The figure shows three views and two pictorial views of one solid part (mm, origin at its lowest corner). Answer the questions. A direction names the side the tool comes from. Round coordinates to 2 decimals unless told otherwise and drop trailing zeros. Order: outer loops, then holes, each group sorted by start corner. A loop starts at its lowest first (then second) coordinate and runs counter-clockwise, first axis right, second up. Notation, with made-up numbers: M 88.25,19.25 L 118.25,19.25 A3 ccw 118.25,23.25 Z; hole C 68,61.25 d1. An arc over 180 degrees is marked long. Return JSON: item names as keys, results as strings.
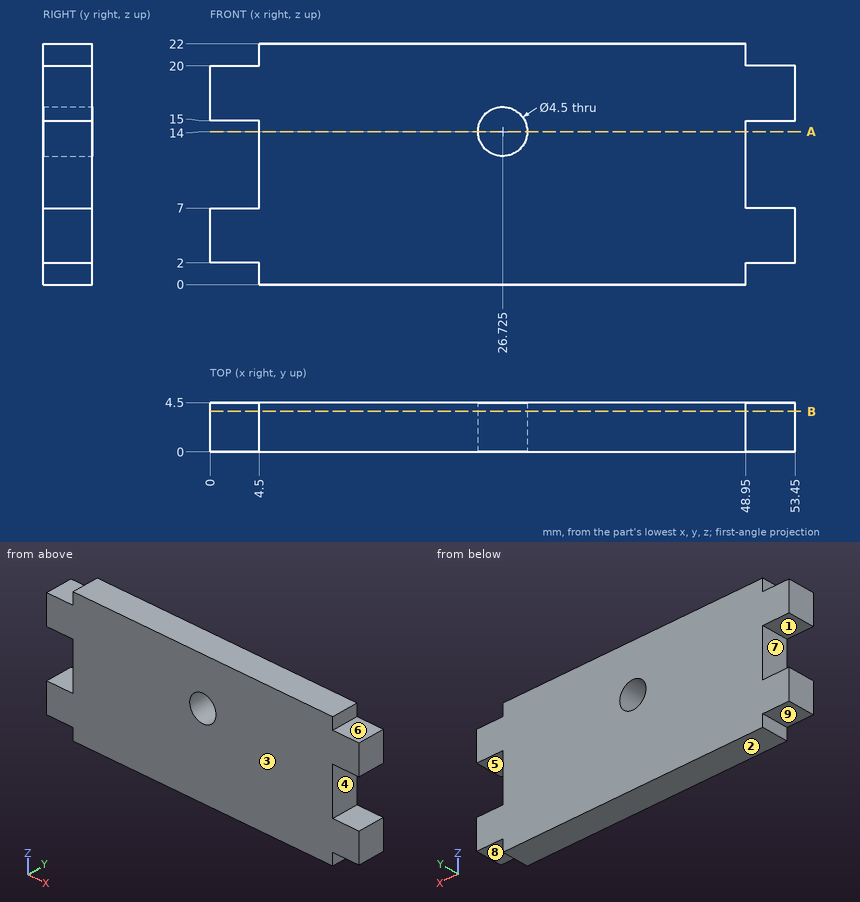
Item 1: Each of these flat-tipped pins is pushed along its axis until it touches: pin 1 (2 mm diameter, centred on x = 51.5, y = 3.5, fed in from -Z); pin 2 (0.6 mm diameter, centred on y = 2, z = 21, fed in from +X); pin 3 (5 mm diameter, centred on x = 26.725, z = 14, fed in from +Y); pin 4 (0.6 mm diameter, centred on y = 2, z = 20.5, fed in from -X). Where does it stop, or does it pass through?
Output:
{"pin 1": "stops at z = 2", "pin 2": "stops at x = 48.95", "pin 3": "stops at y = 4.5", "pin 4": "stops at x = 4.5"}
Item 2: Find section A-A (z = 14). Determine the outline of the cut face in (x, y) (3 decimals).
Output:
{"outline": "M 4.5,0 L 24.475,0 L 24.475,4.5 L 4.5,4.5 Z; M 28.975,0 L 48.95,0 L 48.95,4.5 L 28.975,4.5 Z"}
Item 3: Find section B-B (y = 3.7). Determine the outline of the cut face in (x, z) (3 decimals), plus the area to 3 significant figures.
Output:
{"outline": "M 0,2 L 4.5,2 L 4.5,0 L 48.95,0 L 48.95,2 L 53.45,2 L 53.45,7 L 48.95,7 L 48.95,15 L 53.45,15 L 53.45,20 L 48.95,20 L 48.95,22 L 4.5,22 L 4.5,20 L 0,20 L 0,15 L 4.5,15 L 4.5,7 L 0,7 Z; hole C 26.725,14 d4.5", "area": "1,050 mm^2"}
Item 4: Consider line 1 along Z through (x, y) = (50, 1.15); line 2 along X through (y, z) = (3.05, 14) (3 decimals); line 3 along Z through (x, y) = (28.5, 3.9). Determine where each line is inside the solid, lowest interval first. Write a range as [from, to].
Output:
{"line 1": "z = [2, 7], [15, 20]", "line 2": "x = [4.5, 24.475], [28.975, 48.95]", "line 3": "z = [0, 12.62], [15.38, 22]"}
Item 5: Which of the six approach directions +Z, -Z, +X, -X, +Y, -Y give full straight-line access (tool end or side, diameter ignored) to the marked faces 5, 6, 7, 8 and 9?
Output:
{"face 5": "+X, +Y, -Y", "face 6": "+Z, +X, +Y, -Y", "face 7": "-X, +Y, -Y", "face 8": "-Z, +X, +Y, -Y", "face 9": "-Z, -X, +Y, -Y"}
Item 6: The mould has two halves that part along Z. Classify the marked faces 1, 2, 3 and 4: pulls with the +Z half, pulls with the -Z half, needs draft (parallel to the pull), parting line crosses it, or undercut.
Output:
{"face 1": "undercut", "face 2": "pulls with the -Z half", "face 3": "needs draft", "face 4": "undercut"}
